Here's the drawing with two shaded views (mm, measured from the low corner). I have some questions. A direction names the side the tool comes from. Round coordinates to 2 decimals unless told otherwise and drop trailing zeros. Order: outer loops, then holes, each group sorted by start corner. A loop starts at its lowest first (then second) coordinate and runs counter-clockwise, first axis right, second up. Notation, with made-up numbers: (84, -24) - (97, -24) arc R5 cw to (97, -16) - close; hole circle Ø1 at (-12, -20). An arc over 180 degrees is marked (long way). Return JSON: item names as keys, results as strings. Group by question number.
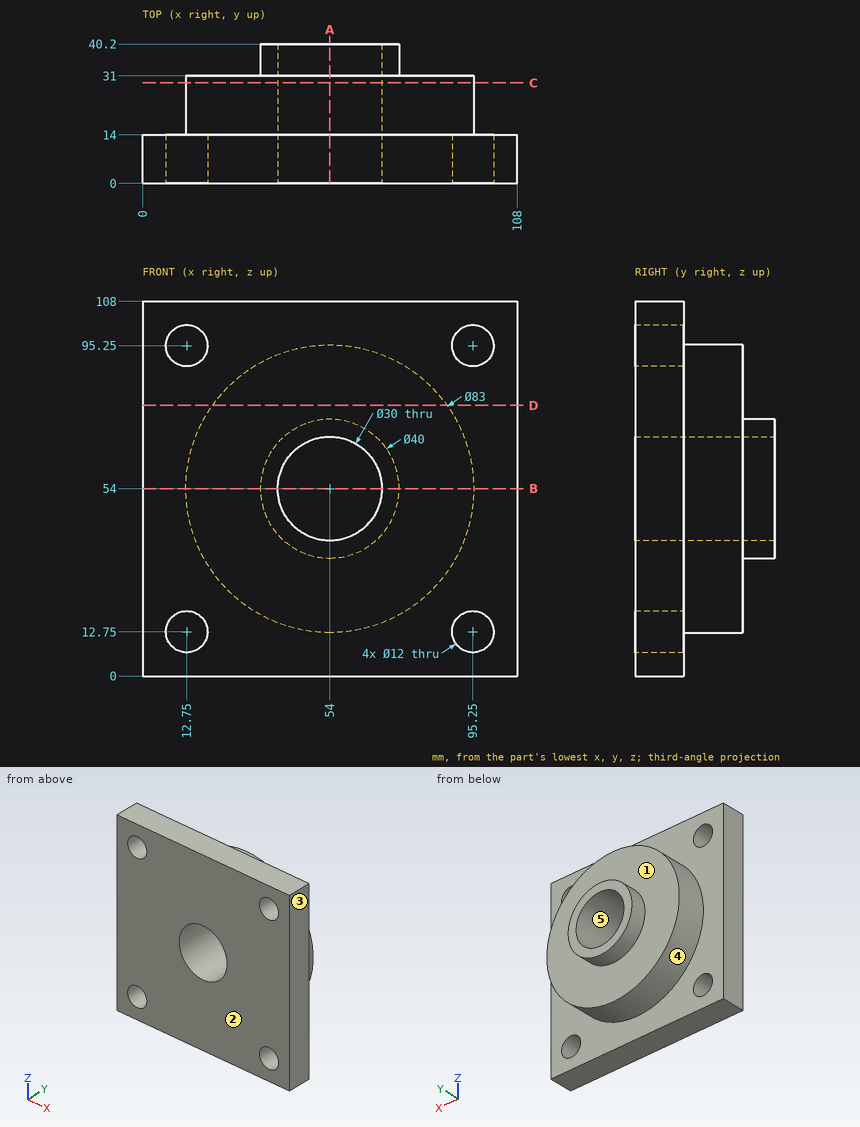
1) I want a section at A-A, the plane x = 54. List the corners of the cut face in (y, z) for me, plus the area to 4 significant figures.
2) If I drill on line 1 along X through (y, z) = (7.5, 95.25); line 2 along Z through (x, y) = (95, 3); line 3 along X through (y, z) = (22, 54), over which ranges is the centre line in solid material (lowest first)? Write a range as from..to.
3) I want a section at D-D, the plane z = 78. List the corners of the cut face in (x, y) for me, plus the area to 3 significant figures.
4) I want a section at C-C, the plane y = 29. List the corners of the cut face in (x, z) for me, plus the area to 3 significant figures.
5) Will these pins go through, and if not, where does the flat tip stop? pin 1 (11 mm diameter, centred on x = 95.25, z = 12.75, fed in from -Y); pin 2 (10 mm diameter, centred on y = 28.5, z = 90, fed in from +X); pin 3 (3 mm diameter, centred on x = 53, y = 25.5, fed in from -Z); pin 4 (6 mm diameter, centred on y = 23.5, z = 91.5, fed in from +X).
6) We'd pull the mould along X, two halves only. Please class the marked faces 3, 4 and 5: +X half, -X half, draft (parallel to the pull), parting line (faces both ways), or undercut.
7) I want a section at B-B, the plane z = 54. List the corners of the cut face in (x, y) for me, plus the area to 4 significant figures.
8) For the marked faces 1 and 2, which set-ups out of +Z, -Z, +X, -X, +Y, -Y let a thin tool reach every point of the face, with its end or its side?
Outcome:
{
 "1": {"outline": "(0, 0) - (14, 0) - (14, 12.5) - (31, 12.5) - (31, 34) - (40.2, 34) - (40.2, 39) - (0, 39) - close; (0, 69) - (40.2, 69) - (40.2, 74) - (31, 74) - (31, 95.5) - (14, 95.5) - (14, 108) - (0, 108) - close", "area": "2,085 mm^2"},
 "2": {"line 1": "0..6.75, 18.75..89.25, 101.25..108", "line 2": "0..6.76, 18.74..89.26, 101.24..108", "line 3": "12.5..39, 69..95.5"},
 "3": {"outline": "(0, 0) - (108, 0) - (108, 14) - (87.86, 14) - (87.86, 31) - (20.14, 31) - (20.14, 14) - (0, 14) - close", "area": "2,660 mm^2"},
 "4": {"outline": "circle Ø83 at (54, 54); hole circle Ø30 at (54, 54)", "area": "4,700 mm^2"},
 "5": {"pin 1": "through", "pin 2": "x = 81.59", "pin 3": "z = 12.5", "pin 4": "x = 77.07"},
 "6": {"face 3": "+X half", "face 4": "parting line", "face 5": "undercut"},
 "7": {"outline": "(0, 0) - (39, 0) - (39, 40.2) - (34, 40.2) - (34, 31) - (12.5, 31) - (12.5, 14) - (0, 14) - close; (69, 0) - (108, 0) - (108, 14) - (95.5, 14) - (95.5, 31) - (74, 31) - (74, 40.2) - (69, 40.2) - close", "area": "2,085 mm^2"},
 "8": {"face 1": "+Y", "face 2": "+Z, -Z, +X, -X, -Y"}
}
